```python
from build123d import *

# Parameters (mm, degrees)
BOSS_EXTRUDE1_DEPTH = 72
FILLET1_R           = 10
SKETCH2_W           = 10
SKETCH2_H           = 20
CUT_EXTRUDE1_DEPTH  = 72
SKETCH3_R           = 18
SKETCH3_R_2         = 9
BOSS_EXTRUDE2_DEPTH = 18
BOSS_EXTRUDE4_DEPTH = 5
RIB20_REACH         = 189.115
SKETCH6_WALL_W      = 472.375598612
SKETCH6_WALL_H      = 10
RIB21_REACH         = 189.115
SKETCH7_WALL_W      = 445.62728217
SKETCH7_WALL_H      = 10
SKETCH8_R           = 6
CUT_EXTRUDE2_DEPTH  = 100


with BuildPart() as part:
    # Sketch1 → Boss-Extrude1 (new body)
    with BuildSketch(Plane.XY):
        with BuildLine():
            Line((76, 0), (76, 10))
            Line((76, 10), (82, 10))
            ThreePointArc((82, 10), (100, 28), (118, 10))
            Line((118, 10), (154, 10))
            Line((154, 10), (154, 20))
            Line((154, 20), (121.817424229, 20))
            ThreePointArc((121.817424229, 20), (100, 34), (78.182575771, 20))
            Line((78.182575771, 20), (0, 20))
            Line((0, 20), (0, 0))
            Line((0, 0), (76, 0))
        make_face()
    extrude(amount=BOSS_EXTRUDE1_DEPTH)

    # Fillet1
    fillet1_edges = [part.edges().sort_by_distance(p)[0] for p in [
        (154, 15, 0),
        (0, 10, 0),
        (154, 15, 72),
        (0, 10, 72),
    ]]
    fillet(fillet1_edges, radius=FILLET1_R)

    # Sketch2 → Cut-Extrude1 (cut)
    with BuildSketch(Plane(origin=(0, 20, 0), x_dir=(1, 0, 0), z_dir=(0, 1, 0))):
        with Locations((149, -36)):
            Rectangle(SKETCH2_W, SKETCH2_H)
    extrude(amount=-CUT_EXTRUDE1_DEPTH, mode=Mode.SUBTRACT)



with BuildPart() as body_2:
    # Sketch3 → Boss-Extrude2 (new, symmetric)
    with BuildSketch(Plane.XY.offset(36)):
        with Locations((36, 82)):
            Circle(SKETCH3_R)
        with Locations((36, 82)):
            Circle(SKETCH3_R_2, mode=Mode.SUBTRACT)
    extrude(amount=BOSS_EXTRUDE2_DEPTH, both=True)


with BuildPart() as part_1:
    add(part.part)

    add(body_2.part)  # Boss-Extrude4 merges body 2
    # Sketch4 → Boss-Extrude4 (add, symmetric)
    with BuildSketch(Plane(origin=(36, 0, 0), x_dir=(0, 0, -1), z_dir=(1, 0, 0))):
        Polygon((-54, 54), (-54, 70.710811109), (-18, 70.710811109), (-18, 54), (0, 20), (-72, 20), align=None)
    extrude(amount=BOSS_EXTRUDE4_DEPTH, both=True)

    # Sketch6 wall → Rib20 (add, up to next)
    with BuildSketch(Plane(origin=(82.796156549, 60.902139154, 36), x_dir=(0.709625674032, -0.704578883273, 0), z_dir=(0.704578883273, 0.709625674032, 0)), mode=Mode.PRIVATE) as rib20_sk1:
        Rectangle(SKETCH6_WALL_W, SKETCH6_WALL_H)
    rib20_tool1 = extrude(rib20_sk1.sketch, amount=-RIB20_REACH, mode=Mode.PRIVATE) - part_1.part
    add(rib20_tool1.solids().sort_by_distance((82.796156549, 60.902139154, 36))[0])

    # Sketch7 wall → Rib21 (add, up to next)
    with BuildSketch(Plane(origin=(9.33156562, 53.420381253, 36), x_dir=(0.268931250293, 0.963159375501, 0), z_dir=(-0.963159375501, 0.268931250293, 0)), mode=Mode.PRIVATE) as rib21_sk1:
        Rectangle(SKETCH7_WALL_W, SKETCH7_WALL_H)
    rib21_tool1 = extrude(rib21_sk1.sketch, amount=-RIB21_REACH, mode=Mode.PRIVATE) - part_1.part
    add(rib21_tool1.solids().sort_by_distance((9.33156562, 53.420381253, 36))[0])

    # Sketch8 → Cut-Extrude2 (cut)
    with BuildSketch(Plane(origin=(0, 0, 0), x_dir=(1, 0, 0), z_dir=(0, 1, 0))):
        with Locations((64, -18)):
            Circle(SKETCH8_R)
        with Locations((64, -54)):
            Circle(SKETCH8_R)
    extrude(amount=CUT_EXTRUDE2_DEPTH, mode=Mode.SUBTRACT)


solid = part_1.part
```
Design review of the part built by this model. Coordinates are the model's own, in mm. A direction names the side the tool comes from. Round coordinates to 2 decimals unless told otherwise and drop trailing zeros. Write each loop counter-clockwise with the first axis right and the second up, starting at its lowest first coordinate (ties: lowest second). Pieces come first, ordered by that corner, then holes. Notation, with made-up numbers: (65, 56) -> (95, 56) arc R30 cw to (95, 94) -> close; hole circle Ø5 at (-40, 61). An arc over 180 degrees is marked (long way). Answer in a Markdown table with one row per item.
Q1. Take a section at D-D, the plane x = 64. State the section outline as (y, z) points.
The answers:
| item | result |
|---|---|
| outline | (0, 0) -> (20, 0) -> (20, 12) -> (0, 12) -> close; (0, 24) -> (20, 24) -> (20, 31) -> (79.56, 31) -> (79.56, 41) -> (20, 41) -> (20, 48) -> (0, 48) -> close; (0, 60) -> (20, 60) -> (20, 72) -> (0, 72) -> close |
Q2. Draft analysis for pull direction Z (two halves, no side actions). For faces 1 (the face through (144, 15, 36)), 2 (the face through (100, 28, 35)), 3 (the face through (149, 15, 46)), 4 (the face through (151.15, 15.07, 3.01)), state which applies: +Z half, -Z half, draft (parallel to the pull), parting line (faces both ways), or undercut.
The answers:
| item | result |
|---|---|
| face 1 | undercut |
| face 2 | draft |
| face 3 | undercut |
| face 4 | -Z half |
Q3. To check wall thickness, follow L1, parallel to Z at x = 64, y = 9.75; L2, parallel to X at y = 10.75, z = 54; L3, parallel to Y at x = 36, z = 31.5. State the ranges of each line that lie inside material, in increasing order. Write a range as [from, to].
The answers:
| item | result |
|---|---|
| L1 | [0, 12], [24, 48], [60, 72] |
| L2 | [0, 58], [70, 82.02], [117.98, 154] |
| L3 | [0, 73], [91, 100] |
Q4. Take a section at C-C, the plane y = 82. State the section outline as (x, z) points.
The answers:
| item | result |
|---|---|
| outline | (17.31, 31) -> (18, 31) -> (18, 18) -> (27, 18) -> (27, 54) -> (18, 54) -> (18, 41) -> (17.31, 41) -> close; (45, 18) -> (54, 18) -> (54, 31) -> (61.55, 31) -> (61.55, 41) -> (54, 41) -> (54, 54) -> (45, 54) -> close |
Q5. Take a section at B-B, the plane z = 43. State the section outline as (x, y) points, then the cut area to 3 significant figures.
The answers:
| item | result |
|---|---|
| outline | (0, 0) -> (76, 0) -> (76, 10) -> (82, 10) arc R18 cw to (118, 10) -> (144, 10) -> (144, 20) -> (121.82, 20) arc R24 ccw to (78.18, 20) -> (41, 20) -> (41, 64.71) arc R18 ccw (long way) to (31, 64.71) -> (31, 20) -> (0, 20) -> close; hole circle Ø18 at (36, 82) |
| area | 3,340 mm² |
Q6. Take a section at A-A, the plane x = 36. State the section outline as (y, z) points.
The answers:
| item | result |
|---|---|
| outline | (0, 0) -> (20, 0) -> (54, 18) -> (73, 18) -> (73, 54) -> (54, 54) -> (20, 72) -> (0, 72) -> close; (91, 18) -> (100, 18) -> (100, 54) -> (91, 54) -> close |
Q7. For faces 5 (the face through (100, 34, 43)), 6 (the face through (18, 42, 31)), 7 (the face through (36, 37, 63)), list the 3-axis set-ups (+Z, -Z, +X, -X, +Y, -Y) from which the entire face can be reached by the end or side of a thin tool; tool diameter is ignored.
The answers:
| item | result |
|---|---|
| face 5 | +Y |
| face 6 | -Z, -X |
| face 7 | +Z, -X, +Y |
Q8. Clearance check with flat-ended pins moving along their axes: pin 1 Ø1.5 at (x, y) = (95.5, 39.5) entering from +Z; pin 2 Ø8 at (y, z) = (86, 30.5) entering from -X; pin 3 Ø20.5 at (x, y) = (36, 82) entering from -Z. State where each tip first meets the part, or that it passes through.
The answers:
| item | result |
|---|---|
| pin 1 | z = 41 |
| pin 2 | x = 17.32 |
| pin 3 | z = 18 |
